Design review of the part built by this model. Coordinates are the model's own, in mm. A direction names the side the tool comes from. Coordinates: 2 decimals unless noted, no trailing zeros. Loops run counter-clockwise (first coordinate to the right, second up) from the corner with the lowest first, then second, coordinate; pieces in that order, holes last. Notation, with made-up numbers: (18.25, -25.75) -> (67.25, -25.75) arc R24 cw to (67.25, -1.75) -> close; hole circle Ø2 at (17, -37.5). An arc over 180 degrees is marked (long way). Use CSV: the item, a comma, the result in double quotes.
Autodesk Inventor part; units mm, degrees
ref_plane "YZ Plane" through (0, 0, 0) normal (1, 0, 0) x (0, 1, 0)
ref_plane "XZ Plane" through (0, 0, 0) normal (0, 1, 0) x (-1, 0, 0)
ref_plane "XY Plane" through (0, 0, 0) normal (0, 0, 1) x (1, 0, 0)
sketch "Base" plane through (0, 0, 0) normal (0, 0, 1) x (1, 0, 0)
  circle A0 centre (6.3437, -0.0043) radius 44.7044
  line L0 (-53.391, 43.8831) -> (3.4518, 87.3031)
  line L1 (3.4518, 87.3031) -> (126.7242, 46.1195)
  line L2 (21.9665, -51.542) -> (-11.8651, -109.4379)
  line L3 (134.9457, -71.4872) -> (143.2137, -54.1334)
  line L4 (44.7126, -49.2622) -> (124.7112, -76.8356)
  line L5 (44.7126, -49.2622) -> (21.9665, -51.542)
  line L6 (126.7242, 46.1195) -> (143.2137, -54.1334)
  line L7 (134.9457, -71.4872) -> (124.7112, -76.8356)
  line L8 (-30.3614, -103.0627) -> (-11.8651, -109.4379)
  line L9 (-30.3614, -103.0627) -> (-19.8027, -31.8971)
  circle A1 centre (113.0613, -42.5954) radius 19.05 construction
  line L10 (-54.6035, 18.8674) -> (-53.391, 43.8831)
  line L11 (-54.6035, 18.8674) -> (-19.8027, -31.8971)
  line L12 (-94.1669, 0) -> (182.7771, 0) construction
  circle A2 centre (6.3437, -0.0043) radius 3.175
  circle A3 centre (113.0613, -42.5954) radius 3.175
  line L13 (126.7242, 46.1195) -> (-19.8027, -31.8971) construction
  line L14 (3.4518, 87.3031) -> (33.3396, -50.4021) construction
  line L15 (-53.9972, 31.3753) -> (126.7242, 46.1195) construction
  line L16 (134.969, -4.007) -> (-37.2031, -6.5149) construction
  line L17 (-21.1132, -106.2503) -> (39.5241, 75.2519) construction
  line L18 (78.4642, -60.8955) -> (78.4642, 62.2425) construction
  line L19 (21.9665, -51.542) -> (126.7242, 46.1195) construction
  line L20 (0, 0) -> (-53.391, 43.8831) construction
  circle A4 centre (-20.3518, 21.9373) radius 3.175
  circle A5 centre (6.3437, -0.0043) radius 34.5555 construction
  circle A6 centre (-26.006, -12.1525) radius 3.175
  circle A7 centre (0.6895, -34.0941) radius 3.175
  circle A8 centre (33.0392, -21.9459) radius 3.175
  circle A9 centre (38.6934, 12.1439) radius 3.175
  circle A10 centre (11.9979, 34.0855) radius 3.175
  line L21 (113.2722, 38.9571) -> (102.0622, 32.9885) construction
  line L22 (111.78, 41.7596) -> (100.57, 35.791)
  line L23 (103.5543, 30.186) -> (114.7644, 36.1546)
  arc A11 (114.7644, 36.1546) -> (111.78, 41.7596) centre (113.2722, 38.9571) ccw
  arc A12 (100.57, 35.791) -> (103.5543, 30.186) centre (102.0622, 32.9885) ccw
  line L24 (119.5611, -4.2314) -> (106.8611, -4.2314) construction
  line L25 (119.5611, -1.0564) -> (106.8611, -1.0564)
  line L26 (106.8611, -7.4064) -> (119.5611, -7.4064)
  arc A13 (119.5611, -7.4064) -> (119.5611, -1.0564) centre (119.5611, -4.2314) ccw
  arc A14 (106.8611, -1.0564) -> (106.8611, -7.4064) centre (106.8611, -4.2314) ccw
  line L27 (6.6843, 72.4098) -> (9.378, 59.9988) construction
  line L28 (3.5815, 71.7364) -> (6.2752, 59.3254)
  line L29 (12.4807, 60.6722) -> (9.787, 73.0833)
  arc A15 (9.787, 73.0833) -> (3.5815, 71.7364) centre (6.6843, 72.4098) ccw
  arc A16 (6.2752, 59.3254) -> (12.4807, 60.6722) centre (9.378, 59.9988) ccw
  line L30 (-16.2839, -91.795) -> (-12.2597, -79.7494) construction
  line L31 (-13.2725, -92.801) -> (-9.2483, -80.7555)
  line L32 (-15.271, -78.7434) -> (-19.2953, -90.7889)
  arc A17 (-19.2953, -90.7889) -> (-13.2725, -92.801) centre (-16.2839, -91.795) ccw
  arc A18 (-9.2483, -80.7555) -> (-15.271, -78.7434) centre (-12.2597, -79.7494) ccw
  line L33 (78.4642, -44.7756) -> (78.4642, -32.0756) construction
  line L34 (75.2892, -44.7756) -> (75.2892, -32.0756)
  line L35 (81.6392, -32.0756) -> (81.6392, -44.7756)
  arc A19 (75.2892, -44.7756) -> (81.6392, -44.7756) centre (78.4642, -44.7756) ccw
  arc A20 (81.6392, -32.0756) -> (75.2892, -32.0756) centre (78.4642, -32.0756) ccw
  line L36 (-42.4258, 32.3193) -> (-29.7679, 33.352) construction
  line L37 (-42.1676, 29.1548) -> (-29.5097, 30.1875)
  line L38 (-30.0261, 36.5165) -> (-42.684, 35.4838)
  arc A21 (-42.684, 35.4838) -> (-42.1676, 29.1548) centre (-42.4258, 32.3193) ccw
  arc A22 (-29.5097, 30.1875) -> (-30.0261, 36.5165) centre (-29.7679, 33.352) ccw
  line L39 (45.5702, -29.5373) -> (54.8596, -20.8771) construction
  line L40 (47.7352, -31.8596) -> (57.0246, -23.1995)
  line L41 (52.6945, -18.5548) -> (43.4052, -27.2149)
  arc A23 (43.4052, -27.2149) -> (47.7352, -31.8596) centre (45.5702, -29.5373) ccw
  arc A24 (57.0246, -23.1995) -> (52.6945, -18.5548) centre (54.8596, -20.8771) ccw
  point P0 (107.6672, 35.9728)
  point P1 (113.2111, -4.2314)
  point P2 (8.0311, 66.2043)
  point P3 (-14.2718, -85.7722)
  point P4 (78.4642, -38.4256)
  point P5 (-36.0969, 32.8357)
  point P6 (50.2149, -25.2072)
  dimension "d48" = 69.111
  dimension "d0" = 38.1
  dimension "d1" = 89.4088
  dimension "d2" = 55.568
  dimension "d3" = 37.094
  dimension "d4" = 120.3
  dimension "d5" = 81.561
  dimension "d6" = 160.982
  dimension "d7" = 133.392
  dimension "d8" = 143.066
  dimension "d9" = 145.185
  dimension "d10" = 124.151
  dimension "d11" = 130.15
  dimension "d12" = 142.793
  dimension "d13" = 117.814
  dimension "d14" = 19.5642
  dimension "d15" = 25.0158
  dimension "d16" = 71.529
  dimension "d17" = 61.5478
  dimension "d18" = 129.9699
  dimension "d19" = 101.6
  dimension "d20" = 19.2227
  dimension "d21" = 11.5477
  dimension "d22" = 84.6172
  dimension "d23" = 67.056
  dimension "d24" = 22.86
  dimension "d25" = 39.5986
  dimension "d26" = 71.1371
  dimension "d27" = 28.575
  dimension "d28" = 27.8801
  dimension "d29" = 6.35
  dimension "d30" = 6.35
  dimension "d31" = 48.26
  dimension "d32" = 6.35
  dimension "d35" = 360
  dimension "d37" = 6.35
  dimension "d38" = 6.35
  dimension "d39" = 15.24
  dimension "d40" = 12.7
  dimension "d41" = 15.24
  dimension "d43" = 15.24
  dimension "d44" = 15.24
  dimension "d45" = 15.24
  dimension "d46" = 15.7016
  dimension "d49" = 140.583
  dimension "d50" = 4.2314
  dimension "d51" = 91.5631
  dimension "d52" = 12.1439
  dimension "d53" = 0
  dimension "d54" = 30.1875
  dimension "d60" = 126.024
  dimension "d61" = 155.259
extrude "Plate1" add sketch "Base" along normal blind 5.08 contours A0 L9 L11 | A0 L11 L10 L0 L1 L6 L3 L7 L4 L5 L2 L8 L9 | A6 picked at (-0.619, 18.5381)
fillet "Fillet1" radius 6.35 12 edges at (126.7242, 46.1195, 2.54) (3.4518, 87.3031, 2.54) (143.2137, -54.1334, 2.54) (134.9457, -71.4872, 2.54) (124.7112, -76.8356, 2.54) (-11.8651, -109.4379, 2.54) (44.7126, -49.2622, 2.54) (21.9665, -51.542, 2.54) (-30.3614, -103.0627, 2.54) (-19.8027, -31.8971, 2.54) (-54.6035, 18.8674, 2.54) (-53.391, 43.8831, 2.54)
equation "\"d41\" = d39"
equation "\"d43\" = d39"
equation "\"d44\" = d43"
equation "\"d45\" = d43"
equation "\"d47\" = Thickness"
equation "\"BendRadius\" = Thickness"
equation "\"BendReliefWidth\" = Thickness"
equation "\"BendReliefDepth\" = 0.5 * Thickness"
equation "\"CornerReliefSize\" = 4 * Thickness"
equation "\"MinimumRemnant\" = 2 * Thickness"
equation "\"TransitionRadius\" = BendRadius"
equation "\"JacobiRadiusSize\" = BendRadius"
equation "\"GapSize\" = Thickness"
properties part number "UpperLeg2"
Item 1: Add section C-C (z = 1.75). State how many separate pieces and enclosed holes the cut face has, then the cut area to 3 significant figures.
Checked values:
separate pieces,"1"
enclosed holes,"14"
area,"22,600 mm^2"
Item 2: Draft analysis for pull direction Y (two halves, no side actions). For faces 1 (the face through (3.632, 86.485, 2.576)), 2 (the face through (130.14, -74, 2.5)), 3 (the face through (-36.266, 36.007, 2.504)), state which applies: pulls with the +Y half, pulls with the -Y half, needs draft (parallel to the pull), parting line crosses it, or undercut.
Checked values:
face 1,"pulls with the +Y half"
face 2,"pulls with the -Y half"
face 3,"undercut"
Item 3: Clearance check with flat-ended pins moving along their axes: pin 1 (1.5 mm diameter, centred on x = 110.5, z = 2, fed in from -Y); pin 2 (1.5 mm diameter, centred on y = -36, z = 2.5, fed in from -X); pin 3 (2.5 mm diameter, centred on x = 115, z = 1.5, fed in from +Y). State where each tip first meets the part, or that it passes through.
Checked values:
pin 1,"y = -72.2"
pin 2,"x = -20.52"
pin 3,"y = 50.45"
Item 4: To check wall thickness, follow line 1 along X through (y, z) = (-41.5, 3.1); line 2 along X through (y, z) = (-91, 3.6); line 3 along Y through (x, z) = (102.5, 4.7). State the ranges of each line that lie inside material, in increasing order.
Checked values:
line 1,"-21.23 to 75.29, 81.64 to 110.08, 116.04 to 141.14"
line 2,"-28.57 to -19.36, -12.67 to -1.09"
line 3,"-69.18 to 29.84, 36.82 to 54.21"
Item 5: Add section D-D (x = -5). Give the boundary of the cut face in (y, z).
Checked values:
outline,"(-97.69, 0) -> (80.85, 0) -> (80.85, 5.08) -> (-97.69, 5.08) -> close"
Item 6: Add section B-B (x = -37). Give the boundary of the cut face in (y, z), then the cut area to 3 significant figures.
Checked values:
outline,"(-6.81, 0) -> (29.58, 0) -> (29.58, 5.08) -> (-6.81, 5.08) -> close; (35.95, 0) -> (56.4, 0) -> (56.4, 5.08) -> (35.95, 5.08) -> close"
area,"289 mm^2"
Item 7: Machinability: for faces 4 (the face through (-17.255, -84.682, 2.504)), 5 (the face through (34.383, -50.298, 2.504)), 6 (the face through (43, -9, 0)), which of the approach directions +Z, -Z, +X, -X, +Y, -Y give a long, thin tool a straight path to every point of the face, cutting with its end or side? Answer none if there is none.
Checked values:
face 4,"+Z, -Z"
face 5,"+Z, -Z, -Y"
face 6,"-Z, +X, -X, +Y, -Y"
Item 8: Add section A-A (y = -61). Give the boundary of the cut face in (x, z).
Checked values:
outline,"(-24.12, 0) -> (16.44, 0) -> (16.44, 5.08) -> (-24.12, 5.08) -> close; (78.77, 0) -> (139.94, 0) -> (139.94, 5.08) -> (78.77, 5.08) -> close"
